Geometry: final body of the model. Coordinates: model frame, mm. A direction names the side the tool comes from. Give positions to 0.01 mm unless a question says otherwise; leave off trailing zeros. Loops run counter-clockwise (first coordinate to the right, second up) from the corner with the lowest first, then second, coordinate; pieces in that order, holes last. Notation, with made-up numbers: (-40, 67) - (-32, 67) arc R17 ccw to (-32, 72) - close; hole circle Ø5 at (0, 36). An arc over 180 degrees is marked (long way). Use one line per item in the form item = value.
```python
from build123d import *

# Parameters (mm, degrees)
SKETCH1_W            = 20.5
SKETCH1_H            = 9
BOSS_EXTRUDE1_DEPTH  = 6
SKETCH2_W            = 25
SKETCH2_H            = 58
BOSS_EXTRUDE2_DEPTH  = 5
LPATTERN1_COUNT      = 2
LPATTERN1_PITCH      = 49
LPATTERN2_COUNT      = 2
LPATTERN2_PITCH      = 25.5
CUT_EXTRUDE1_REACH   = 62.632
SKETCH3_R            = 2
LPATTERN3_COUNT      = 2
LPATTERN3_PITCH      = 10.3
LPATTERN3_COUNT_DIR2 = 2
LPATTERN3_PITCH_DIR2 = 49
SKETCH4_W            = 25
SKETCH4_H            = 29
BOSS_EXTRUDE3_DEPTH  = 6
LPATTERN4_COUNT      = 2
LPATTERN4_PITCH      = 36.5
SKETCH6_W            = 6
SKETCH6_H            = 29
BOSS_EXTRUDE5_DEPTH  = 46.2
FILLET1_R            = 10
M6_CLEARANCE_HOLE1_D = 6.6
SKETCH9_W            = 6
SKETCH9_H            = 30
BOSS_EXTRUDE6_DEPTH  = 20
BOSS_EXTRUDE7_DEPTH  = 6
LPATTERN5_COUNT      = 2
LPATTERN5_PITCH      = 36.5
FILLET2_R            = 20
M6_CLEARANCE_HOLE2_D = 6.6


with BuildPart() as part:
    # Sketch1 → Boss-Extrude1 (new body)
    with BuildSketch(Plane.XY):
        with Locations((10.25, 4.5)):
            Rectangle(SKETCH1_W, SKETCH1_H)
    boss_extrude1 = extrude(amount=BOSS_EXTRUDE1_DEPTH)

    # Sketch2 → Boss-Extrude2 (add)
    with BuildSketch(Plane(origin=(20.5, 0, 0), x_dir=(0, 0, -1), z_dir=(1, 0, 0))):
        with Locations((6.5, -20)):
            Rectangle(SKETCH2_W, SKETCH2_H)
    boss_extrude2 = extrude(amount=BOSS_EXTRUDE2_DEPTH)

    # LPattern1: Boss-Extrude1 ×2
    with Locations(*[(0, -i * LPATTERN1_PITCH, 0) for i in range(1, LPATTERN1_COUNT)]):
        add(boss_extrude1)

    # LPattern2: Boss-Extrude2 ×2
    with Locations(*[(-i * LPATTERN2_PITCH, 0, 0) for i in range(1, LPATTERN2_COUNT)]):
        add(boss_extrude2)

    # Sketch3 → Cut-Extrude1 (cut, up to next)
    with BuildSketch(Plane.XY.offset(6), mode=Mode.PRIVATE) as cut_extrude1_sk1:
        with Locations((5.1, 4.5)):
            Circle(SKETCH3_R)
    cut_extrude1_tool1 = extrude(cut_extrude1_sk1.sketch, amount=-CUT_EXTRUDE1_REACH, mode=Mode.PRIVATE) & part.part
    cut_extrude1 = cut_extrude1_tool1.solids().sort_by_distance((5.1, 4.5, 6))[0]
    add(cut_extrude1, mode=Mode.SUBTRACT)

    # LPattern3: Cut-Extrude1 2 × 2
    with Locations(*[(i * LPATTERN3_PITCH, -j * LPATTERN3_PITCH_DIR2, 0) for i in range(LPATTERN3_COUNT) for j in range(LPATTERN3_COUNT_DIR2) if (i, j) != (0, 0)]):
        add(cut_extrude1, mode=Mode.SUBTRACT)

    # Sketch4 → Boss-Extrude3 (add)
    with BuildSketch(Plane(origin=(25.5, 0, 0), x_dir=(0, 0, -1), z_dir=(1, 0, 0))):
        with Locations((6.5, -54.5)):
            Rectangle(SKETCH4_W, SKETCH4_H)
    boss_extrude3 = extrude(amount=BOSS_EXTRUDE3_DEPTH)

    # LPattern4: Boss-Extrude3 ×2
    with Locations(*[(-i * LPATTERN4_PITCH, 0, 0) for i in range(1, LPATTERN4_COUNT)]):
        add(boss_extrude3)

    # Sketch6 → Boss-Extrude5 (add)
    with BuildSketch(Plane.XY.offset(6)):
        with Locations((28.5, -54.5)):
            Rectangle(SKETCH6_W, SKETCH6_H)
        with Locations((-8, -54.5)):
            Rectangle(SKETCH6_W, SKETCH6_H)
    extrude(amount=BOSS_EXTRUDE5_DEPTH)

    # Fillet1
    # the kernel refuses this fillet: 10 mm, written as the material it adds along each edge
    with BuildSketch(Plane(origin=(25.5, -40, 6), x_dir=(0, 1, 0), z_dir=(0, 0, -1))) as fillet1_piece_1:
        with BuildLine():
            CenterArc((9.16515139, 10), FILLET1_R, 203.578178478, 66.421821522)
            Line((0, 6), (0, 0))
            Line((0, 0), (9.16515139, 0))
        make_face()
    extrude(amount=25)
    with BuildSketch(Plane(origin=(-5, -40, 6), x_dir=(-1, 0, 0), z_dir=(0, 0, -1))) as fillet1_piece_2:
        with BuildLine():
            CenterArc((10, 9.16515139), FILLET1_R, 180, 66.421821522)
            Line((0, 9.16515139), (0, 0))
            Line((0, 0), (6, 0))
        make_face()
    extrude(amount=25)

    # M6 Clearance Hole1 (through all)
    with Locations(Plane.ZY.offset(11)):
        with Locations((37.2, -55)):
            Hole(M6_CLEARANCE_HOLE1_D / 2)

    # Sketch9 → Boss-Extrude6 (add)
    with BuildSketch(Plane.XZ.offset(69)):
        with Locations((28.5, 37.2)):
            Rectangle(SKETCH9_W, SKETCH9_H)
        with Locations((-8, 37.2)):
            Rectangle(SKETCH9_W, SKETCH9_H)
    extrude(amount=BOSS_EXTRUDE6_DEPTH)

    # Sketch10 → Boss-Extrude7 (add)
    with BuildSketch(Plane(origin=(31.5, 0, 0), x_dir=(0, 0, -1), z_dir=(1, 0, 0))):
        Polygon((-22.2, -80.626229403), (-22.2, -89), (19, -69), (-19.89821605, -69), align=None)
        Polygon((-22.2, -69), (-22.2, -80.626229403), (-19.89821605, -69), align=None)
    boss_extrude7 = extrude(amount=-BOSS_EXTRUDE7_DEPTH)

    # LPattern5: Boss-Extrude7 ×2
    with Locations(*[(-i * LPATTERN5_PITCH, 0, 0) for i in range(1, LPATTERN5_COUNT)]):
        add(boss_extrude7)

    # Fillet2
    fillet2_edges = [part.edges().sort_by_distance(p)[0] for p in [
        (28.5, -40, 52.2),
        (-8, -40, 52.2),
        (28.5, -89, 52.2),
        (-8, -89, 52.2),
    ]]
    fillet(fillet2_edges, radius=FILLET2_R)

    # M6 Clearance Hole2 (through all)
    with Locations(Plane(origin=(31.5, 0, 0), x_dir=(0, 0, -1), z_dir=(1, 0, 0))):
        with Locations((-37.2, -75)):
            Hole(M6_CLEARANCE_HOLE2_D / 2)


solid = part.part
```
(1) Pin query (flat end, axial travel): P1, Ø5.5, axis at y = -75, z = 37.2, coming from the +X side; P2, Ø8, axis at x = 12, y = -39, coming from the +Z side; P3, Ø3, axis at y = -72, z = 36.5, coming from the +X side; P4, Ø5, axis at x = 15, z = 3, coming from the -Y side. Return the tip coordinate at first contact, or that it passes through.
Solution:
P1 = through
P2 = 6
P3 = 31.5
P4 = -49
(2) Material intervals for L1, parallel to Y at x = 5.1, z = 2.05; L2, parallel to X at y = -67, z = 11; L3, parallel to Y at x = 30, z = 37.2, sorted ascending. Write a range as from..to.
Solution:
L1 = -49..-46.5, -42.5..-40, 0..2.5, 6.5..9
L2 = -11..-5, 25.5..31.5
L3 = -88.36..-78.3, -71.7..-58.3, -51.7..-40.64
(3) Cut plane D-D (x = 27). Return the cut outline in (y, z), plus the area to 3 significant figures.
Solution:
outline = (-89, 22.2) - (-69, -19) - (-36.1, -19) - (-36.1, 6) - (-40, 6) - (-40, 32.2) arc R20 ccw to (-60, 52.2) - (-69, 52.2) arc R20 ccw to (-89, 32.2) - close; hole circle Ø6.6 at (-75, 37.2); hole circle Ø6.6 at (-55, 37.2)
area = 2,930 mm2
(4) Access query for faces 1 (the face through (7, -49, 2)), 2 (the face through (10, 0, 3)), 3 (the face through (25.5, -64, 17)), 4 (the face through (0, -20, -6)). Directions: +Z, -Z, +X, -X, +Y, -Y. A direction counts if a zero-diameter tool reaches every point of the face in a straight line with its end or side. Return the directions, or none.
Solution:
face_1 = +Z, -Z, -Y
face_2 = +Z, -Z
face_3 = +Z, -Y
face_4 = -Z
(5) Pull-direction query (X, two-part tool) for faces 5 (the face through (25.5, -11, -6)), 6 (the face through (28, -40, 19)), 7 (the face through (17.247, 3.734, 3.042)); classes: released by +X, released by -X, zero draft, split by the parting line, or undercut.
Solution:
face_5 = released by +X
face_6 = zero draft
face_7 = undercut
(6) Cut plane C-C (x = 11). Return the cut outline in (y, z).
Solution:
outline = (-49, 0) - (-40, 0) - (-40, 6) - (-49, 6) - close; (0, 0) - (9, 0) - (9, 6) - (0, 6) - close
(7) Cut plane A-A (y = 4.5). Return the cut outline in (x, z).
Solution:
outline = (-5, -19) - (0, -19) - (0, 0) - (3.1, 0) - (3.1, 6) - (-5, 6) - close; (7.1, 0) - (13.4, 0) - (13.4, 6) - (7.1, 6) - close; (17.4, 0) - (20.5, 0) - (20.5, -19) - (25.5, -19) - (25.5, 6) - (17.4, 6) - close
(8) Cut plane B-B (z = 23.5). Return the cut outline in (x, y), plus the area to 3 significant figures.
Solution:
outline = (-11, -89) - (-5, -89) - (-5, -40) - (-11, -40) - close; (25.5, -89) - (31.5, -89) - (31.5, -40) - (25.5, -40) - close
area = 588 mm2
